Check sheet for the modelled part. Datum: model origin and axes. Units: mm. Round coordinates to 2 decimals unless told otherwise and drop trailing zeros. Write each loop counter-clockwise with the first axis right and the second up, starting at its lowest first coordinate (ties: lowest second). Pieces come first, ordered by that corner, then holes. Notation, with made-up numbers: M -36.5,-23 L 21.5,-23 A12 cw 21.5,-11 Z; hole C -11,-33 d3. An arc over 180 degrees is marked long. Answer in a Markdown table with one row per item.
```python
from build123d import *

# Parameters (mm, degrees)
SKETCH1_W               = 60
SKETCH1_H               = 60
SKETCH1_R               = 1.65
BOSS_EXTRUDE1_DEPTH     = 4
SKETCH2_R               = 2.15
BOSS_EXTRUDE2_DEPTH     = 4
FILLET1_R               = 10
FILLET2_R               = 3
CUT_EXTRUDE1_DEPTH      = 70.081473638
CUT_EXTRUDE1_DEPTH_BACK = 70.081473638
SKETCH3_W               = 25
SKETCH3_H               = 25
FILLET3_R               = 3


with BuildPart() as part:
    # Sketch1 → Boss-Extrude1 (new body)
    with BuildSketch(Plane(origin=(0, 0, 0), x_dir=(1, 0, 0), z_dir=(0, 1, 0))):
        Rectangle(SKETCH1_W, SKETCH1_H)
        with Locations(Location((-24.5, 24.5, 0), (0, 0, 270))):
            Circle(SKETCH1_R, mode=Mode.SUBTRACT)
        with Locations(Location((24.5, 24.5, 0), (0, 0, 270))):
            Circle(SKETCH1_R, mode=Mode.SUBTRACT)
        with Locations(Location((-24.5, -24.5, 0), (0, 0, 270))):
            Circle(SKETCH1_R, mode=Mode.SUBTRACT)
        with Locations(Location((24.5, -24.5, 0), (0, 0, 270))):
            Circle(SKETCH1_R, mode=Mode.SUBTRACT)
    extrude(amount=BOSS_EXTRUDE1_DEPTH)

    # Sketch2 → Boss-Extrude2 (add)
    with BuildSketch(Plane(origin=(0, 4, 0), x_dir=(1, 0, 0), z_dir=(0, 1, 0))):
        with BuildLine():
            Line((-37.5, 50), (37.5, 50))
            ThreePointArc((37.5, 50), (47.5, 40), (37.5, 30))
            Line((37.5, 30), (-37.5, 30))
            ThreePointArc((-37.5, 30), (-47.5, 40), (-37.5, 50))
        make_face()
        with Locations(Location((-37.5, 40, 0), (0, 0, 270))):
            Circle(SKETCH2_R, mode=Mode.SUBTRACT)
        with Locations(Location((37.5, 40, 0), (0, 0, 270))):
            Circle(SKETCH2_R, mode=Mode.SUBTRACT)
    extrude(amount=-BOSS_EXTRUDE2_DEPTH)

    # Fillet1
    # the kernel refuses this fillet: 10 mm, written as the material it adds along each edge
    with BuildSketch(Plane(origin=(-30, 0, -30), x_dir=(-0.9999598282483387, 0, -0.008963363740972157), z_dir=(0, 1, 0))) as fillet1_piece_1:
        with BuildLine():
            CenterArc((9.911370685, 9.932373054), FILLET1_R, 180.51356979, 82.819244219)
            Line((-0.088227598, 9.842739417), (-1.088187426, 9.833776053))
            Line((-1.088187426, 9.833776053), (-0.999959828, -0.008963364))
            Line((-0.999959828, -0.008963364), (0.008963364, -0.999959828))
            ThreePointArc((0.008963364, -0.999959828), (7.508662076, -0.9327346), (8.6342496, -0.993237305))
            Line((8.6342496, -0.993237305), (8.750351517, 0))
        make_face()
    extrude(amount=4)
    with BuildSketch(Plane(origin=(30, 0, -30), x_dir=(0.9999598282483387, 0, -0.008963363740972154), z_dir=(0, 1, 0))) as fillet1_piece_2:
        with BuildLine():
            CenterArc((9.911370685, -9.932373054), FILLET1_R, 96.667185992, 82.819244219)
            Line((-0.088227598, -9.842739417), (-1.088187426, -9.833776053))
            Line((-1.088187426, -9.833776053), (-0.999959828, 0.008963364))
            Line((-0.999959828, 0.008963364), (0.008963364, 0.999959828))
            ThreePointArc((0.008963364, 0.999959828), (7.508662076, 0.9327346), (8.6342496, 0.993237305))
            Line((8.6342496, 0.993237305), (8.750351517, 0))
        make_face()
    extrude(amount=4)
    # the kernel refuses this fillet: 10 mm, written as the material it takes off along each edge

    # Fillet2
    fillet2_edges = [part.edges().sort_by_distance(p)[0] for p in [
        (30, 2, 30),
        (-30, 2, 30),
    ]]
    fillet(fillet2_edges, radius=FILLET2_R)

    # Sketch3 → Cut-Extrude1 (cut, two sides: drawn at the far end of the back side and taken through both)
    with BuildSketch(Plane(origin=(0, 4, 0), x_dir=(1, 0, 0), z_dir=(0, 1, 0)).offset(-CUT_EXTRUDE1_DEPTH_BACK)):
        Rectangle(SKETCH3_W, SKETCH3_H)
    extrude(amount=CUT_EXTRUDE1_DEPTH + CUT_EXTRUDE1_DEPTH_BACK, mode=Mode.SUBTRACT)

    # Fillet3
    fillet3_edges = [part.edges().sort_by_distance(p)[0] for p in [
        (12.5, 2, -12.5),
        (12.5, 2, 12.5),
        (-12.5, 2, 12.5),
        (-12.5, 2, -12.5),
    ]]
    fillet(fillet3_edges, radius=FILLET3_R)


solid = part.part
```
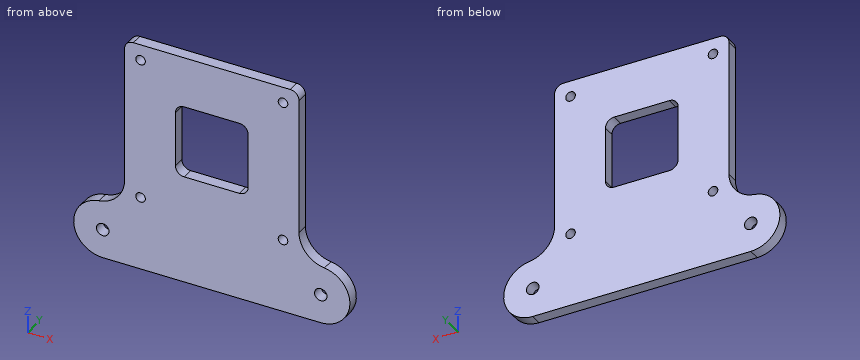
1. Section check D-D, the plane z = 20. Record the cut outline in (x, y), and give its area (3 significant figures).
Found:
| item | result |
|---|---|
| outline | M -30,0 L 30,0 L 30,4 L -30,4 Z |
| area | 240 mm2 |
2. Section check A-A, the plane z = -40. Record the cut outline in (x, y), and give its area (3 significant figures).
Found:
| item | result |
|---|---|
| outline | M -47.5,0 L -39.65,0 L -39.65,4 L -47.5,4 Z; M -35.35,0 L 35.35,0 L 35.35,4 L -35.35,4 Z; M 39.65,0 L 47.5,0 L 47.5,4 L 39.65,4 Z |
| area | 346 mm2 |
3. Go/stop test with flat-tipped pins: pin 1 (4 mm diameter, centred on x = -37.5, z = -40, fed in from +Y); pin 2 (2 mm diameter, centred on y = 3, z = 4.5, fed in from -X); pin 3 (12 mm diameter, centred on x = 16.5, z = 12, fed in from -Y); pin 4 (1.5 mm diameter, centred on y = 2.5, z = -28, fed in from -X). Record where each tip stops, or that it passes through.
Found:
| item | result |
|---|---|
| pin 1 | passes through |
| pin 2 | stops at x = -30 |
| pin 3 | stops at y = 0 |
| pin 4 | stops at x = -34.89 |
4. Section check B-B, the plane x = 24.5. Record the cut outline in (y, z).
Found:
| item | result |
|---|---|
| outline | M 0,-50 L 4,-50 L 4,-26.15 L 0,-26.15 Z; M 0,-22.85 L 4,-22.85 L 4,22.85 L 0,22.85 Z; M 0,26.15 L 4,26.15 L 4,30 L 0,30 Z |
5. Section check C-C, the plane y = 3.15. Record the cut outline in (x, z).
Found:
| item | result |
|---|---|
| outline | M -38.75,-30.08 A10 ccw -37.5,-50 L 37.5,-50 A10 ccw 38.75,-30.08 A10 cw 30,-20.16 L 30,27 A3 ccw 27,30 L -27,30 A3 ccw -30,27 L -30,-20.16 A10 cw Z; hole C -37.5,-40 d4.3; hole C -24.5,-24.5 d3.3; hole C -24.5,24.5 d3.3; hole M -12.5,-9.5 A3 ccw -9.5,-12.5 L 9.5,-12.5 A3 ccw 12.5,-9.5 L 12.5,9.5 A3 ccw 9.5,12.5 L -9.5,12.5 A3 ccw -12.5,9.5 Z; hole C 24.5,-24.5 d3.3; hole C 24.5,24.5 d3.3; hole C 37.5,-40 d4.3 |
6. Scan lines: L1, parallel to X at y = 2.6, z = -40; L2, parallel to X at y = 1.9, z = 24.5; L3, parallel to X at y = 2.95, z = 1.5. Record each from-to range of solid material in increasing order.
Found:
| item | result |
|---|---|
| L1 | x = -47.5 to -39.65, -35.35 to 35.35, 39.65 to 47.5 |
| L2 | x = -30 to -26.15, -22.85 to 22.85, 26.15 to 30 |
| L3 | x = -30 to -12.5, 12.5 to 30 |
